from build123d import *

# Parameters (mm, degrees)
SKETCH1_W               = 6.35
SKETCH1_H               = 50.8
SKETCH1_W_2             = 12.7
SKETCH1_H_2             = 25.4
SKETCH1_W_3             = 25.4
SKETCH1_H_3             = 3.175
CUT_EXTRUDE1_DEPTH      = 114.858173839
CUT_EXTRUDE1_DEPTH_BACK = 114.858173839
SKETCH2_W               = 25.4
SKETCH2_H               = 25.4


with BuildPart() as part:
    # Sketch1 → Revolve1 (revolve)
    with BuildSketch(Plane(origin=(0, 0, 0), x_dir=(1, 0, 0), z_dir=(0, 1, 0))):
        with Locations((0, 50.8)):
            Rectangle(SKETCH1_W, SKETCH1_H)
        with Locations((0, 12.7)):
            Rectangle(SKETCH1_W_2, SKETCH1_H_2)
        with Locations((0, 77.7875)):
            Rectangle(SKETCH1_W_3, SKETCH1_H_3)
    revolve(axis=Axis((6.35, 0, 0), (-1, 0, 0)))

    # Sketch2 → Cut-Extrude1 (cut, two sides: drawn at the far end of the back side and taken through both)
    with BuildSketch(Plane(origin=(6.35, 0, 0), x_dir=(0, 0, -1), z_dir=(1, 0, 0)).offset(-CUT_EXTRUDE1_DEPTH_BACK)):
        Rectangle(SKETCH2_W, SKETCH2_H)
    extrude(amount=CUT_EXTRUDE1_DEPTH + CUT_EXTRUDE1_DEPTH_BACK, mode=Mode.SUBTRACT)


solid = part.part
Input: part model. Units: mm. Frame: model coordinates. A direction names the side the tool comes from. Give positions to 0.01 mm unless a question says otherwise; leave off trailing zeros. Write each loop counter-clockwise with the first axis right and the second up, starting at its lowest first coordinate (ties: lowest second). Pieces come first, ordered by that corner, then holes. Notation, with made-up numbers: M 70.5,55 L 82.5,55 A20 cw 82.5,63 Z; hole C 37.5,-36 d9. An arc over 180 degrees is marked long. Write item = value, one per line. Start each with the question number.
1) Reachability of faces 1 (the cylindrical face through (8.004, 46.367, 60.47)), 2 (the cylindrical face through (-7.871, 46.367, 60.47)), 3 (the flat face through (0, 0, -12.7)), 4 (the flat face through (-12.7, -30, -71)) from +Z, -Z, +X, -X, +Y, -Y: full face, straight path, thin tool, end or side. Return the list, or none.
2) Draft query along Z for faces 5 (the flat face through (12.7, -30, -71)), 6 (the cylindrical face through (0.18, -23.84, -75.71)), 7 (the flat face through (-6.35, 17, 0)), 8 (the flat face through (0, -12.7, 0)). Return one class per face: +Z half, -Z half, draft (parallel to the pull), parting line (faces both ways), or undercut.
3) Cut plane C-C on x = 0.5. Return the cut outline in (y, z) (3 decimals), then the cut area to 3 significant figures.
4) Cut plane D-D on z = 17. Return the cut outline in (x, y) (3 decimals), then the cut area to 3 significant figures.
5) First-contact query: pin 1 Ø6.5 at (x, y) = (-1, -6) entering from -Z; pin 2 Ø8 at (x, y) = (4.5, -56.5) entering from +Z; pin 3 Ø8 at (x, z) = (-4, -38) entering from -Y. Flat tips, straight axial feed; report the tip coordinate or a pass-through.
6) Material intervals for line 1 along Y through (x, z) = (5.5, 0) (3 decimals); line 2 along Z through (x, y) = (-5.5, 21), sorted ascending. Write a range as [from, to].
7) Cut plane A-A on z = 0. Return the cut outline in (x, y) (3 decimals).
Solved:
q1.face_1 = +X
q1.face_2 = -X
q1.face_3 = +X, -X
q1.face_4 = +Z, -Z, -X, +Y, -Y
q2.face_5 = draft
q2.face_6 = parting line
q2.face_7 = undercut
q2.face_8 = undercut
q3.outline = C 0,0 d158.75; hole M -12.7,-12.7 L 12.7,-12.7 L 12.7,12.7 L -12.7,12.7 Z
q3.area = 19,100 mm2
q4.outline = M -12.7,-77.533 L 12.7,-77.533 L 12.7,-74.279 L 3.175,-74.279 L 3.175,-18.872 L 6.35,-18.872 L 6.35,18.872 L 3.175,18.872 L 3.175,74.279 L 12.7,74.279 L 12.7,77.533 L -12.7,77.533 L -12.7,74.279 L -3.175,74.279 L -3.175,18.872 L -6.35,18.872 L -6.35,-18.872 L -3.175,-18.872 L -3.175,-74.279 L -12.7,-74.279 Z
q4.area = 1,350 mm2
q5.pin_1 = -79.33
q5.pin_2 = 59.53
q5.pin_3 = -71.72
q6.line_1 = [-79.375, -76.2], [-25.4, -12.7], [12.7, 25.4], [76.2, 79.375]
q6.line_2 = [-76.55, -73.25], [-14.29, 14.29], [73.25, 76.55]
q7.outline = M -12.7,-79.375 L 12.7,-79.375 L 12.7,-76.2 L 3.175,-76.2 L 3.175,-25.4 L 6.35,-25.4 L 6.35,-12.7 L -6.35,-12.7 L -6.35,-25.4 L -3.175,-25.4 L -3.175,-76.2 L -12.7,-76.2 Z; M -12.7,76.2 L -3.175,76.2 L -3.175,25.4 L -6.35,25.4 L -6.35,12.7 L 6.35,12.7 L 6.35,25.4 L 3.175,25.4 L 3.175,76.2 L 12.7,76.2 L 12.7,79.375 L -12.7,79.375 Z
